```python
from build123d import *

# Parameters (mm, degrees)
SKETCH1_W           = 12
SKETCH1_H           = 8
BOSS_EXTRUDE1_DEPTH = 3.5
CUT_EXTRUDE1_DEPTH  = 4.5
SKETCH3_W           = 3.5
SKETCH3_H           = 2
BOSS_EXTRUDE2_DEPTH = 13
SKETCH4_W           = 13
SKETCH4_H           = 2
BOSS_EXTRUDE3_DEPTH = 4.5


with BuildPart() as part:
    # Sketch1 → Boss-Extrude1 (new body)
    with BuildSketch(Plane.XY):
        with Locations((6, 4)):
            Rectangle(SKETCH1_W, SKETCH1_H)
    extrude(amount=BOSS_EXTRUDE1_DEPTH)

    # Sketch2 → Cut-Extrude1 (cut, through all)
    with BuildSketch(Plane.XY.offset(3.5)):
        with BuildLine():
            Line((5.25, 5.5), (5.25, 2.5))
            ThreePointArc((5.25, 2.5), (4, 1.25), (2.75, 2.5))
            Line((2.75, 2.5), (2.75, 5.5))
            ThreePointArc((2.75, 5.5), (4, 6.75), (5.25, 5.5))
        make_face()
        with BuildLine():
            Line((10.25, 5.5), (10.25, 2.5))
            ThreePointArc((10.25, 2.5), (9, 1.25), (7.75, 2.5))
            Line((7.75, 2.5), (7.75, 5.5))
            ThreePointArc((7.75, 5.5), (9, 6.75), (10.25, 5.5))
        make_face()
    extrude(amount=-CUT_EXTRUDE1_DEPTH, mode=Mode.SUBTRACT)

    # Sketch3 → Boss-Extrude2 (add)
    with BuildSketch(Plane.ZY):
        with Locations((1.75, 7)):
            Rectangle(SKETCH3_W, SKETCH3_H)
    extrude(amount=BOSS_EXTRUDE2_DEPTH)

    # Sketch4 → Boss-Extrude3 (add)
    with BuildSketch(Plane(origin=(0, 0, 0), x_dir=(-1, 0, 0), z_dir=(0, 0, -1))):
        with Locations((6.5, 7)):
            Rectangle(SKETCH4_W, SKETCH4_H)
    extrude(amount=BOSS_EXTRUDE3_DEPTH)


solid = part.part
```
For this review, take the finished solid that the model builds, in its own axes (mm). A direction names the side the tool comes from. Coordinates: 2 decimals unless noted, no trailing zeros. Loops run counter-clockwise (first coordinate to the right, second up) from the corner with the lowest first, then second, coordinate; pieces in that order, holes last. Notation, with made-up numbers: (26, 22) -> (72, 22) arc R23 ccw to (72, 33) -> close; hole circle Ø7 at (30.25, 65.25). An arc over 180 degrees is marked (long way). Return JSON: item names as keys, results as strings. Group by question number.
(1) For pin 1 Ø2.5 at (y, z) = (3.5, 2.5) entering from -X; pin 2 Ø1.6 at (y, z) = (7, -2) entering from +X; pin 3 Ø1 at (x, y) = (6, 4.5) entering from -Z, all flat-tipped, find the tip position at first contact; note any pin that passes through.
(2) To check wall thickness, follow L1, parallel to X at y = 3.5, z = 1; L2, parallel to X at y = 6.25, z = -3; L3, parallel to Z at x = 1.25, y = 6. State the ranges of each line that lie inside material, in increasing order.
(3) Consider section D-D, the plane y = 6.5. Give the boundary of the cut face in (x, z).
(4) Consider section A-A, the plane y = 3.25. Give the boundary of the cut face in (x, z).
(5) Consider section C-C, the plane x = 4. Give the boundary of the cut face in (y, z), plus the area to 3 significant figures.
(6) Consider section B-B, the plane z = 1. Give the boundary of the cut face in (x, y), plus the area to 3 significant figures.
(7) Tool access review of faces 5 (the flat face through (-6, 6, 0)), 6 (the flat face through (12, 4, 2)), 7 (the cylindrical face through (8.97, 6.75, 1.77)): name each direction out of +Z, -Z, +X, -X, +Y, -Y from which nothing blocks a thin tool from reaching the whole face with its end or side.
(8) Mouldability with a two-part tool opening along X and no side actions: class faces 1 (the flat face through (0, 7, -2)), 2 (the flat face through (6, 4, 0)), 3 (the flat face through (0, 3, 2)), 4 (the flat face through (7.75, 4, 2)) as pulls with the +X half, pulls with the -X half, needs draft (parallel to the pull), parting line crosses it, or undercut.
Results below:
{
 "1": {"pin 1": "stops at x = 0", "pin 2": "stops at x = 0", "pin 3": "stops at z = 0"},
 "2": {"L1": "x = 0 to 2.75, 5.25 to 7.75, 10.25 to 12", "L2": "x = -13 to 0", "L3": "z = 0 to 3.5"},
 "3": {"outline": "(-13, -4.5) -> (0, -4.5) -> (0, 0) -> (3.25, 0) -> (3.25, 3.5) -> (-13, 3.5) -> close; (4.75, 0) -> (8.25, 0) -> (8.25, 3.5) -> (4.75, 3.5) -> close; (9.75, 0) -> (12, 0) -> (12, 3.5) -> (9.75, 3.5) -> close"},
 "4": {"outline": "(0, 0) -> (2.75, 0) -> (2.75, 3.5) -> (0, 3.5) -> close; (5.25, 0) -> (7.75, 0) -> (7.75, 3.5) -> (5.25, 3.5) -> close; (10.25, 0) -> (12, 0) -> (12, 3.5) -> (10.25, 3.5) -> close"},
 "5": {"outline": "(0, 0) -> (1.25, 0) -> (1.25, 3.5) -> (0, 3.5) -> close; (6.75, 0) -> (8, 0) -> (8, 3.5) -> (6.75, 3.5) -> close", "area": "8.75 mm2"},
 "6": {"outline": "(-13, 6) -> (0, 6) -> (0, 0) -> (12, 0) -> (12, 8) -> (-13, 8) -> close; hole (2.75, 2.5) arc R1.25 ccw to (5.25, 2.5) -> (5.25, 5.5) arc R1.25 ccw to (2.75, 5.5) -> close; hole (7.75, 2.5) arc R1.25 ccw to (10.25, 2.5) -> (10.25, 5.5) arc R1.25 ccw to (7.75, 5.5) -> close", "area": "97.2 mm2"},
 "7": {"face 5": "+Z, -Z, -X, -Y", "face 6": "+Z, -Z, +X, +Y, -Y", "face 7": "+Z, -Z"},
 "8": {"face 1": "pulls with the +X half", "face 2": "needs draft", "face 3": "pulls with the -X half", "face 4": "undercut"}
}
